Input: part model. Units: mm. Frame: model coordinates. A direction names the side the tool comes from. Give positions to 0.01 mm unless a question says otherwise; leave off trailing zeros. Write each loop counter-clockwise with the first axis right and the second up, starting at its lowest first coordinate (ties: lowest second). Pieces come first, ordered by that corner, then holes. Notation, with made-up numbers: (-10.5, 29.25) - (45.5, 29.25) arc R7 ccw to (45.5, 35.25) - close; hole circle Ø11 at (17.25, 70). An arc over 180 degrees is marked (long way). Answer as a JSON object with one key per item and string values. Group by question number.
from build123d import *

# Parameters (mm, degrees)
SKETCH1_R           = 4.25
SKETCH1_R_2         = 1.05
BOSS_EXTRUDE1_DEPTH = 23
BOSS_EXTRUDE3_DEPTH = 2
SKETCH4_W           = 21
SKETCH4_H           = 41
CUT_EXTRUDE1_DEPTH  = 50.288548817
BOSS_EXTRUDE4_START = 42
BOSS_EXTRUDE4_DEPTH = 42


with BuildPart() as part:
    # Sketch1 → Boss-Extrude1 (new, symmetric)
    with BuildSketch(Plane.XY):
        with BuildLine():
            Line((-0.798015115, 9.968107738), (11.201984885, 9.968107738))
            ThreePointArc((11.201984885, 9.968107738), (19.90012903, 28.53283063), (7.687881875, 45))
            Line((7.687881875, 45), (3.464101615, 45))
            Line((3.464101615, 45), (0, 47))
            Line((0, 47), (10.5, 47))
            ThreePointArc((10.5, 47), (22.975048867, 25.465576737), (8.550692083, 5.18513885))
            ThreePointArc((8.550692083, 5.18513885), (-4.554689659, -8.902516617), (-0.798015115, 9.968107738))
        make_face()
        Circle(SKETCH1_R, mode=Mode.SUBTRACT)
        with Locations((0, 7)):
            Circle(SKETCH1_R_2, mode=Mode.SUBTRACT)
        with Locations((7, 0)):
            Circle(SKETCH1_R_2, mode=Mode.SUBTRACT)
        with Locations((0, -7)):
            Circle(SKETCH1_R_2, mode=Mode.SUBTRACT)
        with Locations((-7, 0)):
            Circle(SKETCH1_R_2, mode=Mode.SUBTRACT)
    extrude(amount=BOSS_EXTRUDE1_DEPTH, both=True)

    # Sketch3 → Boss-Extrude3 (add)
    with BuildSketch(Plane.XY.offset(23)):
        with BuildLine():
            Line((0, 47), (3.464101615, 45))
            Line((3.464101615, 45), (7.687881875, 45))
            ThreePointArc((7.687881875, 45), (19.90012903, 28.53283063), (11.201984885, 9.968107738))
            Line((11.201984885, 9.968107738), (0, 9.968107738))
            Line((0, 9.968107738), (0, 47))
        make_face()
    boss_extrude3 = extrude(amount=-BOSS_EXTRUDE3_DEPTH)

    # Mirror1: Boss-Extrude3 across plane
    add(boss_extrude3.mirror(Plane.XY))

    # Sketch4 → Cut-Extrude1 (cut, through all)
    with BuildSketch(Plane(origin=(0, 9.968107738, 0), x_dir=(1, 0, 0), z_dir=(0, 1, 0))):
        Rectangle(SKETCH4_W, SKETCH4_H)
    extrude(amount=-CUT_EXTRUDE1_DEPTH, mode=Mode.SUBTRACT)

    # Sketch6 → Boss-Extrude4 (add)
    with BuildSketch(Plane.XY.offset(-21).offset(BOSS_EXTRUDE4_START)):
        with BuildLine():
            Line((0, 22.833916422), (19.654261637, 22.833916422))
            ThreePointArc((19.654261637, 22.833916422), (19.326374482, 21.389653004), (18.892510823, 19.973613057))
            Line((18.892510823, 19.973613057), (0, 19.973613057))
            Line((0, 19.973613057), (0, 22.833916422))
        make_face()
    extrude(amount=-BOSS_EXTRUDE4_DEPTH)


solid = part.part
1) Cut plane B-B on y = 0. Count the separate pieces of the cut face and the enclosed holes in it, and give its area (3 significant figures).
2) Pin query (flat end, axial travel): P1, Ø3, axis at y = 13, z = 15, coming from the -X side; P2, Ø8, axis at x = 5, z = 11.5, coming from the -Y side; P3, Ø2, axis at y = 25, z = -0.5, coming from the -X side. Return the tip coordinate at first contact, or that it passes through.
3) Cut plane C-C on z = 0. Return the cut outline in (x, y).
4) Mould query, pull axis Y, two halves, no side actions, for faces 1 (the face through (-1.05, 7.05, 21.73)), 2 (the face through (10, 25, -23)), 3 (the face through (5, 47, 0)). Classes: +Y half, -Y half, draft (parallel to the pull), parting line (faces both ways), or undercut.
5) Line query: line 1 along X through (y, z) = (0, -22.2); line 2 along Z through (x, y) = (11, 27); line 3 along Y through (x, z) = (12, 1.5). Output: solid intervals per line, ascending. Write a range as from..to.
6) Reachability of faces 4 (the face through (10.5, 8, 0)), 5 (the face through (-8.05, 0.05, 21.73)), 6 (the face through (10, 22.834, 0)) from +Z, -Z, +X, -X, +Y, -Y: full face, straight path, thin tool, end or side. Return the list, or none.
7) Cut plane A-A on x = 7. Return the cut outline in (y, z).
8) Cut plane D-D on y = -7. Return the cut outline in (x, z), and give its area (3 significant figures).
Filled in:
{
 "1": {"separate pieces": "8", "enclosed holes": "0", "area": "36.5 mm²"},
 "2": {"P1": "stops at x = 13.19", "P2": "stops at y = 19.97", "P3": "stops at x = 19.84"},
 "3": {"outline": "(0, 19.97) - (18.89, 19.97) arc R20 cw to (11.2, 9.97) - (10.5, 9.97) - (10.5, 6.07) arc R23 ccw to (10.5, 47) - (0, 47) - (3.46, 45) - (7.69, 45) arc R20 cw to (19.65, 22.83) - (0, 22.83) - close"},
 "4": {"face 1": "undercut", "face 2": "draft", "face 3": "+Y half"},
 "5": {"line 1": "x = -10..-8.05, -5.95..-4.25, 4.25..5.95, 8.05..10", "line 2": "z = -23..-21, 21..23", "line 3": "y = 6.92..10.54, 19.97..22.83, 42.54..46.16"},
 "6": {"face 4": "-X, -Y", "face 5": "+Z, -Z", "face 6": "-X"},
 "7": {"outline": "(-7.14, -23) - (-1.05, -23) - (-1.05, -20.5) - (-7.14, -20.5) - close; (-7.14, 20.5) - (-1.05, 20.5) - (-1.05, 23) - (-7.14, 23) - close; (1.05, -23) - (47, -23) - (47, 23) - (1.05, 23) - (1.05, 20.5) - (9.97, 20.5) - (9.97, 21) - (19.97, 21) - (19.97, -21) - (9.97, -21) - (9.97, -20.5) - (1.05, -20.5) - close; hole (22.83, -21) - (45, -21) - (45, 21) - (22.83, 21) - close"},
 "8": {"outline": "(-7.14, -23) - (-1.05, -23) - (-1.05, -20.5) - (-7.14, -20.5) - close; (-7.14, 20.5) - (-1.05, 20.5) - (-1.05, 23) - (-7.14, 23) - close; (1.05, -23) - (7.14, -23) - (7.14, -20.5) - (1.05, -20.5) - close; (1.05, 20.5) - (7.14, 20.5) - (7.14, 23) - (1.05, 23) - close", "area": "60.9 mm²"}
}
